Geometry: final body of the model. Coordinates: model frame, mm. Face numbers are marked on the shaded views. A direction names the side the tool comes from. Round coordinates to 2 decimals unless told otherwise and drop trailing zeros. Loops run counter-clockwise (first coordinate to the right, second up) from the corner with the lowest first, then second, coordinate; pieces in that order, holes last. Notation, with made-up numbers: (89.25, 71) - (98.25, 71) arc R20 ccw to (98.25, 87) - close; hole circle Ø5 at (78, -17). An arc over 180 degrees is marked (long way). Answer in a Markdown table with one row per item. Add a question column.
from build123d import *

# Parameters (mm, degrees)
BOSS_EXTRUDE1_DEPTH = 300
CUT_EXTRUDE1_DEPTH  = 200
CUT_EXTRUDE2_DEPTH  = 200
SKETCH4_R           = 52.323508973
SKETCH4_W           = 45.776374161
SKETCH4_H           = 79.884183104
BOSS_EXTRUDE2_DEPTH = 200
BOSS_EXTRUDE3_DEPTH = 200


with BuildPart() as part:
    # Sketch1 → Boss-Extrude1 (new body)
    with BuildSketch(Plane.XY):
        Polygon((144.337567297, -250), (288.675134595, 0), (144.337567297, 250), (-144.337567297, 250), (-288.675134595, 0), (-144.337567297, -250), align=None)
    extrude(amount=BOSS_EXTRUDE1_DEPTH)

    # Sketch2 → Cut-Extrude1 (cut)
    with BuildSketch(Plane.XY.offset(300)):
        Polygon((254.034118443, 0), (127.017059222, 220), (-127.017059222, 220), (-254.034118443, 0), (-127.017059222, -220), (127.017059222, -220), align=None)
    extrude(amount=-CUT_EXTRUDE1_DEPTH, mode=Mode.SUBTRACT)

    # Sketch3 → Cut-Extrude2 (cut)
    with BuildSketch(Plane.XY.offset(300)):
        Polygon((-127.017059222, -220), (-144.337567297, -250), (-253.098126512, -358.157726196), (520.522562071, -384.900169752), (552.995529246, 34.383141715), (288.675134595, 0), (254.034118443, 0), align=None)
    extrude(amount=-CUT_EXTRUDE2_DEPTH, mode=Mode.SUBTRACT)

    # Sketch4 → Boss-Extrude2 (add)
    with BuildSketch(Plane.XY.offset(100)):
        with Locations((71.000041779, 65.908432745)):
            Circle(SKETCH4_R)
        with Locations((-104.985312432, 70.865886515)):
            Rectangle(SKETCH4_W, SKETCH4_H)
    extrude(amount=BOSS_EXTRUDE2_DEPTH)

    # Sketch5 → Boss-Extrude3 (add)
    with BuildSketch(Plane.XY.offset(100)):
        Polygon((46.793412905, -127.30955218), (5.420185833, -85.764472901), (-51.245521762, -100.822198942), (-66.538002284, -157.425004263), (-25.164775212, -198.970083543), (31.500932383, -183.912357501), align=None)
    extrude(amount=BOSS_EXTRUDE3_DEPTH)


solid = part.part
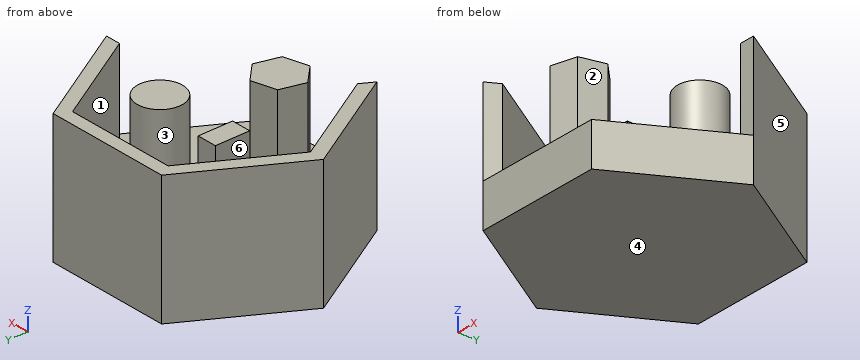
1) Section A-A, the plane x = -98. Return the cut outline in (y, z), and give its area (3 significant figures).
2) Section D-D, the plane z = 83. Return the cut outline in (x, y).
3) Pull-direction query (Y, two-part tool) for the marked faces 4, 5 and 6; classes: pulls with the +Y half, pulls with the -Y half, needs draft (parallel to the pull), parting line crosses it, or undercut.
4) Section B-B, the plane z = 238. Return the cut outline in (x, y) (1 decimal), and give its area (3 significant figures).
5) Section C-C, the plane y = 197. Return the cut outline in (x, z), and give its area (3 significant figures).
6) Reachability of the marked faces 1, 2 and 3 from +Z, -Z, +X, -X, +Y, -Y: full face, straight path, thin tool, end or side. Return the list, or none.
7) Contact query for flat-ended pins moving along their axis: pin 1 Ø8 at (y, z) = (75, 170) entering from -X; pin 2 Ø2 at (y, z) = (184.5, 259.5) entering from -X; pin 3 Ø23 at (x, z) = (-108.5, 161) entering from -Y. Output: stop coordinate, or through.
8) Material intervals for line 1 along X through (y, z) = (26, 163); line 2 along Y through (x, z) = (-83.5, 285.5); line 3 along Z through (x, y) = (-59, -74.5), sorted ascending. Write a range as from..to.
Evaluation:
| question | item | result |
|---|---|---|
| 1 | outline | (-250, 0) - (250, 0) - (250, 300) - (220, 300) - (220, 100) - (110.81, 100) - (110.81, 300) - (30.92, 300) - (30.92, 100) - (-250, 100) - close |
| 1 | area | 72,000 mm² |
| 2 | outline | (-288.68, 0) - (-144.34, -250) - (144.34, -250) - (288.68, 0) - (144.34, 250) - (-144.34, 250) - close |
| 3 | face 4 | needs draft |
| 3 | face 5 | pulls with the +Y half |
| 3 | face 6 | undercut |
| 4 | outline | (-288.7, 0) - (-144.3, -250) - (-127, -220) - (-254, 0) - (-127, 220) - (127, 220) - (254, 0) - (288.7, 0) - (144.3, 250) - (-144.3, 250) - close; (-127.9, 30.9) - (-82.1, 30.9) - (-82.1, 110.8) - (-127.9, 110.8) - close; (-66.5, -157.4) - (-25.2, -199) - (31.5, -183.9) - (46.8, -127.3) - (5.4, -85.8) - (-51.2, -100.8) - close; circle Ø104.6 at (71, 65.9) |
| 4 | area | 53,800 mm² |
| 5 | outline | (-174.94, 0) - (174.94, 0) - (174.94, 300) - (140.3, 300) - (140.3, 100) - (-140.3, 100) - (-140.3, 300) - (-174.94, 300) - close |
| 5 | area | 48,800 mm² |
| 6 | face 1 | +Z, -Y |
| 6 | face 2 | +Z, +X, -Y |
| 6 | face 3 | +Z |
| 7 | pin 1 | stops at x = -247.68 |
| 7 | pin 2 | stops at x = -182.73 |
| 7 | pin 3 | stops at y = 30.92 |
| 8 | line 1 | x = -273.66..-239.02, 37.16..104.84, 239.02..273.66 |
| 8 | line 2 | y = 30.92..110.81, 220..250 |
| 8 | line 3 | z = 0..100 |
